Here's how the part is built. I have some questions about the finished solid (model axes, mm). Give positions to 0.01 mm unless a question says otherwise; leave off trailing zeros. Write each loop counter-clockwise with the first axis right and the second up, starting at its lowest first coordinate (ties: lowest second). Pieces come first, ordered by that corner, then holes. Notation, with made-up numbers: M -10.75,-10.5 L 19.25,-10.5 A15 cw 19.25,16.5 Z; hole C -17.75,-2.75 d11. An arc over 180 degrees is marked long. Use one line per item in the form item = value. Start each with the question number.
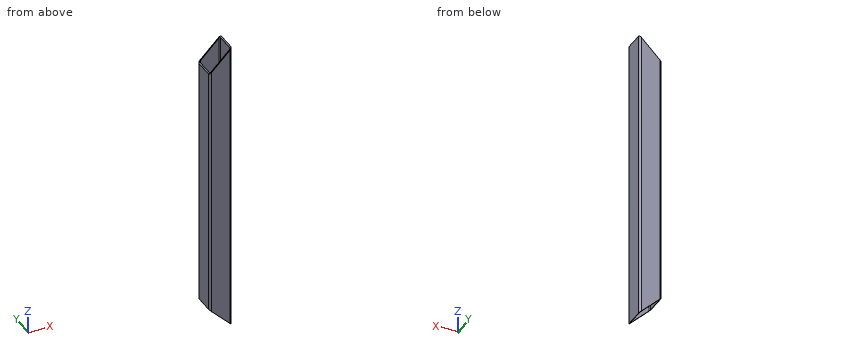
Autodesk Inventor part; units mm, degrees
ref_plane "Start plane" through (0, 0, -17.5) normal (0, 0, 1) x (1, 0, 0)
ref_plane "End plane" through (0, 0, 447.5) normal (0, 0, 1) x (1, 0, 0)
ref_plane "Work Plane5" through (17.5, 0, 447.5) normal (-0.7071, 0, 0.7071) x (0.7071, 0, 0.7071)
ref_plane "Start plane" through (0, 0, -17.5) normal (0, 0, 1) x (1, 0, 0)
ref_plane "End plane" through (0, 0, 447.5) normal (0, 0, 1) x (1, 0, 0)
sketch "Sketch" plane through (0, 0, 0) normal (0, 0, 1) x (1, 0, 0)
  line L0 (-17.5, -14.3) -> (-17.5, 14.3)
  line L1 (-14.3, 17.5) -> (14.3, 17.5)
  line L2 (17.5, 14.3) -> (17.5, -14.3)
  line L3 (14.3, -17.5) -> (-14.3, -17.5)
  arc A0 (-17.5, -14.3) -> (-14.3, -17.5) centre (-14.3, -14.3) ccw
  arc A1 (-14.3, 17.5) -> (-17.5, 14.3) centre (-14.3, 14.3) ccw
  arc A2 (17.5, 14.3) -> (14.3, 17.5) centre (14.3, 14.3) ccw
  arc A3 (14.3, -17.5) -> (17.5, -14.3) centre (14.3, -14.3) ccw
  arc A4 (-14.3, 15.9) -> (-15.9, 14.3) centre (-14.3, 14.3) ccw
  line L4 (-14.3, 15.9) -> (14.3, 15.9)
  arc A5 (15.9, 14.3) -> (14.3, 15.9) centre (14.3, 14.3) ccw
  line L5 (15.9, 14.3) -> (15.9, -14.3)
  arc A6 (14.3, -15.9) -> (15.9, -14.3) centre (14.3, -14.3) ccw
  line L6 (14.3, -15.9) -> (-14.3, -15.9)
  arc A7 (-15.9, -14.3) -> (-14.3, -15.9) centre (-14.3, -14.3) ccw
  line L7 (-15.9, -14.3) -> (-15.9, 14.3)
  line L8 (0, 25.4278) -> (0, -25.4278) construction
  line L9 (-25.4278, 0) -> (25.4278, 0) construction
  dimension "d7" = 3.2
  dimension "d10" = 35
  dimension "d11" = 35
  dimension "d12" = 1.6
  dimension "d15" = 17.5
  dimension "d16" = 17.5
extrude "Body" add sketch "Sketch" along normal up to surface (465 mm away) from surface at -17.5
sketch "Sketch3" plane through (0, 0, 0) normal (0, 0, 1) x (1, 0, 0)
  line L0 (0, 0) -> (10, 0)
ref_plane "Work Plane3" through (0, 0, 0) normal (0, -1, 0) x (1, 0, 0)
sketch "Sketch4" plane through (0, 0, 0) normal (0, -1, 0) x (1, 0, 0)
  line L0 (-2, -17.5) -> (12, -17.5)
  line L1 (-2, 447.5) -> (12, 447.5)
  dimension "d18" = 465
ref_plane "Work Plane5" through (17.5, 0, 447.5) normal (-0.7071, 0, 0.7071) x (0.7071, 0, 0.7071)
split "Split2" plane through (17.5, 0, 447.5) removes the side toward (-0.7071, 0, 0.7071)
ref_plane "Work Plane12" through (0, 180, -17.5) normal (0, 0, -1) x (-1, 0, 0)
split "Split6" plane through (0, 180, -17.5) removes the side toward (0, 0, -1)
ref_plane "Work Plane13" through (17.5, 0, -17.5) normal (-0.7071, 0, -0.7071) x (-0.7071, 0, 0.7071)
split "Split7" plane through (17.5, 0, -17.5) removes the side toward (-0.7071, 0, -0.7071)
equation "\"d7\" = G_IR"
equation "\"d10\" = G_H"
equation "\"d11\" = G_W"
equation "\"d12\" = G_T"
equation "\"d15\" = 0.5 * d10"
equation "\"d16\" = 0.5 * d11"
equation "\"d3\" = G_L"
equation "\"G_W\" = 35"
equation "\"G_H\" = 35"
equation "\"G_T\" = 1.6"
equation "\"G_IR\" = 3.2"
equation "\"G_L\" = d18"
equation "\"G_OFFSET_START\" = 17.5"
equation "\"G_OFFSET_END\" = 17.5"
equation "\"d13\" = -G_OFFSET_START"
equation "\"d14\" = G_OFFSET_END + B_L"
properties part number "AS 1163 - C350L0 35x35x1.6 SHS - 465" material "Steel, Mild"
1) Suppose I cut it at C-C, the plane y = -0.5. List the corners of the cut face in (x, z) for me.
2) Suppose I cut it at A-A, the plane x = 7. List the corners of the cut face in (y, z) for me, and give its area (3 significant figures).
3) Please list where these lines run through material, in increasing order: line 1 (X direction, y = 9.5, z = 28); line 2 (Y direction, x = 15.5, z = 135.5).
4) Suppose I cut it at B-B, the plane z = 63.5. List the corners of the cut face in (x, y) for me.
Checks:
q1.outline = M -17.5,17.5 L -15.9,15.9 L -15.9,414.1 L -17.5,412.5 Z; M 15.9,-15.9 L 17.5,-17.5 L 17.5,447.5 L 15.9,445.9 Z
q2.outline = M -17.5,-7 L -15.9,-7 L -15.9,437 L -17.5,437 Z; M 15.9,-7 L 17.5,-7 L 17.5,437 L 15.9,437 Z
q2.area = 1,420 mm^2
q3.line_1 = -17.5 to -15.9, 15.9 to 17.5
q3.line_2 = -17.27 to -15.36, 15.36 to 17.27
q4.outline = M -17.5,-14.3 A3.2 ccw -14.3,-17.5 L 14.3,-17.5 A3.2 ccw 17.5,-14.3 L 17.5,14.3 A3.2 ccw 14.3,17.5 L -14.3,17.5 A3.2 ccw -17.5,14.3 Z; hole M -15.9,-14.3 A1.6 ccw -14.3,-15.9 L 14.3,-15.9 A1.6 ccw 15.9,-14.3 L 15.9,14.3 A1.6 ccw 14.3,15.9 L -14.3,15.9 A1.6 ccw -15.9,14.3 Z
